The listing builds one solid part. Answer for the finished solid, in the listing's coordinates (mm). A direction names the side the tool comes from. Give positions to 0.01 mm unless a question says otherwise; leave off trailing zeros. Loops run counter-clockwise (first coordinate to the right, second up) from the corner with the lowest first, then second, coordinate; pieces in that order, holes last. Notation, with made-up numbers: (-9.5, -19.5) - (4.5, -19.5) arc R19 cw to (4.5, -4.5) - close; hole circle Ø10 at (29.25, 16). An arc over 180 degrees is marked (long way). Write each question's results on one line, items separated by ' | '.
from build123d import *
from OCP.BRepFilletAPI import BRepFilletAPI_MakeChamfer

# Parameters (mm, degrees)
SKETCH1_W           = 225
SKETCH1_H           = 190
SKETCH1_R           = 2.65
BOSS_EXTRUDE1_DEPTH = 5
BOSS_EXTRUDE2_DEPTH = 5
CHAMFER1_SIZE       = 8.660254038
CHAMFER1_SIZE_2     = 5


with BuildPart() as part:
    # Sketch1 → Boss-Extrude1 (new body)
    with BuildSketch(Plane(origin=(0, 0, 0), x_dir=(1, 0, 0), z_dir=(0, 1, 0))):
        with Locations((112.5, 95)):
            Rectangle(SKETCH1_W, SKETCH1_H)
        with Locations(Location((10, 180, 0), (0, 0, 270))):
            Circle(SKETCH1_R, mode=Mode.SUBTRACT)
        with Locations(Location((40, 180, 0), (0, 0, 270))):
            Circle(SKETCH1_R, mode=Mode.SUBTRACT)
        with Locations(Location((185, 180, 0), (0, 0, 270))):
            Circle(SKETCH1_R, mode=Mode.SUBTRACT)
        with Locations(Location((215, 180, 0), (0, 0, 270))):
            Circle(SKETCH1_R, mode=Mode.SUBTRACT)
        with Locations(Location((215, 10, 0), (0, 0, 90))):
            Circle(SKETCH1_R, mode=Mode.SUBTRACT)
        with Locations(Location((185, 10, 0), (0, 0, 90))):
            Circle(SKETCH1_R, mode=Mode.SUBTRACT)
        with Locations(Location((40, 10, 0), (0, 0, 90))):
            Circle(SKETCH1_R, mode=Mode.SUBTRACT)
        with Locations(Location((10, 10, 0), (0, 0, 90))):
            Circle(SKETCH1_R, mode=Mode.SUBTRACT)
    extrude(amount=BOSS_EXTRUDE1_DEPTH)

    # Sketch2 → Boss-Extrude2 (add)
    with BuildSketch(Plane(origin=(0, 5, 0), x_dir=(1, 0, 0), z_dir=(0, 1, 0))):
        with BuildLine():
            Line((51.576473623, 139.026400418), (167.040167682, 43.276019978))
            ThreePointArc((167.040167682, 43.276019978), (174.080636831, 43.933130432), (173.423526377, 50.973599582))
            Line((173.423526377, 50.973599582), (57.959832318, 146.723980022))
            ThreePointArc((57.959832318, 146.723980022), (50.919363169, 146.066869568), (51.576473623, 139.026400418))
        make_face()
    boss_extrude2 = extrude(amount=BOSS_EXTRUDE2_DEPTH)

    # Mirror1: Boss-Extrude2 across plane
    add(boss_extrude2.mirror(Plane(origin=(0, 0, -95), x_dir=(1, 0, 0), z_dir=(0, 0, -1))))

    # Chamfer1
    chamfer1_edges_1 = [part.edges().sort_by_distance(p)[0] for p in [
        (139.770083841, 5, -65.890235846),
    ]]
    chamfer1_side_1 = [part.faces().sort_by_distance(p)[0] for p in [
        (139.706250254, 5, -65.81326005),
    ]]
    chamfer1_edges_2 = [part.edges().sort_by_distance(p)[0] for p in [
        (174.080636831, 5, -43.933130432),
    ]]
    chamfer1_side_2 = [part.faces().sort_by_distance(p)[0] for p in [
        (174.157612628, 5, -43.869296845),
    ]]
    chamfer1_edges_3 = [part.edges().sort_by_distance(p)[0] for p in [
        (146.878196714, 5, -72.986799791),
    ]]
    chamfer1_side_3 = [part.faces().sort_by_distance(p)[0] for p in [
        (146.942030301, 5, -73.063775587),
    ]]
    chamfer1_edges_4 = [part.edges().sort_by_distance(p)[0] for p in [
        (146.878196714, 5, -117.013200209),
    ]]
    chamfer1_side_4 = [part.faces().sort_by_distance(p)[0] for p in [
        (146.942030301, 5, -116.936224413),
    ]]
    chamfer1_edges_5 = [part.edges().sort_by_distance(p)[0] for p in [
        (174.080636831, 5, -146.066869568),
    ]]
    chamfer1_side_5 = [part.faces().sort_by_distance(p)[0] for p in [
        (174.157612628, 5, -146.130703155),
    ]]
    chamfer1_edges_6 = [part.edges().sort_by_distance(p)[0] for p in [
        (139.770083841, 5, -124.109764154),
    ]]
    chamfer1_side_6 = [part.faces().sort_by_distance(p)[0] for p in [
        (139.706250254, 5, -124.18673995),
    ]]
    chamfer1_edges_7 = [part.edges().sort_by_distance(p)[0] for p in [
        (85.229916159, 5, -124.109764154),
    ]]
    chamfer1_side_7 = [part.faces().sort_by_distance(p)[0] for p in [
        (85.293749746, 5, -124.18673995),
    ]]
    chamfer1_edges_8 = [part.edges().sort_by_distance(p)[0] for p in [
        (85.229916159, 5, -65.890235846),
    ]]
    chamfer1_side_8 = [part.faces().sort_by_distance(p)[0] for p in [
        (85.293749746, 5, -65.81326005),
    ]]
    chamfer1_edges_9 = [part.edges().sort_by_distance(p)[0] for p in [
        (50.919363169, 5, -146.066869568),
    ]]
    chamfer1_side_9 = [part.faces().sort_by_distance(p)[0] for p in [
        (50.842387372, 5, -146.130703155),
    ]]
    chamfer1_edges_10 = [part.edges().sort_by_distance(p)[0] for p in [
        (50.919363169, 5, -43.933130432),
    ]]
    chamfer1_side_10 = [part.faces().sort_by_distance(p)[0] for p in [
        (50.842387372, 5, -43.869296845),
    ]]
    chamfer1_edges_11 = [part.edges().sort_by_distance(p)[0] for p in [
        (78.121803286, 5, -117.013200209),
    ]]
    chamfer1_side_11 = [part.faces().sort_by_distance(p)[0] for p in [
        (78.057969699, 5, -116.936224413),
    ]]
    chamfer1_edges_12 = [part.edges().sort_by_distance(p)[0] for p in [
        (78.121803286, 5, -72.986799791),
    ]]
    chamfer1_side_12 = [part.faces().sort_by_distance(p)[0] for p in [
        (78.057969699, 5, -73.063775587),
    ]]
    chamfer1 = BRepFilletAPI_MakeChamfer(part.part.solid().wrapped)
    for e in chamfer1_edges_1:
        chamfer1.Add(CHAMFER1_SIZE - 0.0001, CHAMFER1_SIZE_2 - 0.0001, e.wrapped, chamfer1_side_1[0].wrapped)
    for e in chamfer1_edges_2:
        chamfer1.Add(CHAMFER1_SIZE - 0.0001, CHAMFER1_SIZE_2 - 0.0001, e.wrapped, chamfer1_side_2[0].wrapped)
    for e in chamfer1_edges_3:
        chamfer1.Add(CHAMFER1_SIZE - 0.0001, CHAMFER1_SIZE_2 - 0.0001, e.wrapped, chamfer1_side_3[0].wrapped)
    for e in chamfer1_edges_4:
        chamfer1.Add(CHAMFER1_SIZE - 0.0001, CHAMFER1_SIZE_2 - 0.0001, e.wrapped, chamfer1_side_4[0].wrapped)
    for e in chamfer1_edges_5:
        chamfer1.Add(CHAMFER1_SIZE - 0.0001, CHAMFER1_SIZE_2 - 0.0001, e.wrapped, chamfer1_side_5[0].wrapped)
    for e in chamfer1_edges_6:
        chamfer1.Add(CHAMFER1_SIZE - 0.0001, CHAMFER1_SIZE_2 - 0.0001, e.wrapped, chamfer1_side_6[0].wrapped)
    for e in chamfer1_edges_7:
        chamfer1.Add(CHAMFER1_SIZE - 0.0001, CHAMFER1_SIZE_2 - 0.0001, e.wrapped, chamfer1_side_7[0].wrapped)
    for e in chamfer1_edges_8:
        chamfer1.Add(CHAMFER1_SIZE - 0.0001, CHAMFER1_SIZE_2 - 0.0001, e.wrapped, chamfer1_side_8[0].wrapped)
    for e in chamfer1_edges_9:
        chamfer1.Add(CHAMFER1_SIZE - 0.0001, CHAMFER1_SIZE_2 - 0.0001, e.wrapped, chamfer1_side_9[0].wrapped)
    for e in chamfer1_edges_10:
        chamfer1.Add(CHAMFER1_SIZE - 0.0001, CHAMFER1_SIZE_2 - 0.0001, e.wrapped, chamfer1_side_10[0].wrapped)
    for e in chamfer1_edges_11:
        chamfer1.Add(CHAMFER1_SIZE - 0.0001, CHAMFER1_SIZE_2 - 0.0001, e.wrapped, chamfer1_side_11[0].wrapped)
    for e in chamfer1_edges_12:
        chamfer1.Add(CHAMFER1_SIZE - 0.0001, CHAMFER1_SIZE_2 - 0.0001, e.wrapped, chamfer1_side_12[0].wrapped)
    add(Compound.cast(chamfer1.Shape()), mode=Mode.REPLACE)  # a hair under: the kernel refuses the full size


solid = part.part
Item 1: A cutting plane is placed at A-A, the plane z = -180. Determine the outline of the cut face in (x, y).
Values found:
outline: (0, 0) - (7.35, 0) - (7.35, 5) - (0, 5) - close; (12.65, 0) - (37.35, 0) - (37.35, 5) - (12.65, 5) - close; (42.65, 0) - (182.35, 0) - (182.35, 5) - (42.65, 5) - close; (187.65, 0) - (212.35, 0) - (212.35, 5) - (187.65, 5) - close; (217.65, 0) - (225, 0) - (225, 5) - (217.65, 5) - close
Item 2: Find the intervals of material crossed by line 1 along X through (y, z) = (2.35, -10); line 2 along Z through (x, y) = (215, 1.15); line 3 along Y through (x, z) = (176, -162), in increasing order. Write a range as [from, to].
Values found:
line 1: x = [0, 7.35], [12.65, 37.35], [42.65, 182.35], [187.65, 212.35], [217.65, 225] | line 2: z = [-190, -182.65], [-177.35, -12.65], [-7.35, 0] | line 3: y = [0, 5]
Item 3: A cutting plane is placed at C-C, the plane y = 8. Determine the outline of the cut face in (x, z).
Values found:
outline: (49.37, -136.36) arc R8.46 ccw to (60.17, -149.39) - (112.5, -106) - (164.83, -149.39) arc R8.46 ccw to (175.63, -136.36) - (125.76, -95) - (175.63, -53.64) arc R8.46 ccw to (164.83, -40.61) - (112.5, -84) - (60.17, -40.61) arc R8.46 ccw to (49.37, -53.64) - (99.24, -95) - close
Item 4: Flat-ended cylindrical pins translate along their axes: P1, Ø5, axis at x = 215, z = -180, coming from the +Y side; P2, Ø7, axis at x = 215, z = -10, coming from the +Y side; P3, Ø6, axis at x = 185, z = -180, coming from the -Y side. Find the tip coordinate at first contact, or state that the pin passes through.
Values found:
P1: passes through | P2: stops at y = 5 | P3: stops at y = 0
Item 5: A cutting plane is placed at B-B, the plane x = 215. Determine the outline of the cut face in (y, z).
Values found:
outline: (0, -190) - (5, -190) - (5, -182.65) - (0, -182.65) - close; (0, -177.35) - (5, -177.35) - (5, -12.65) - (0, -12.65) - close; (0, -7.35) - (5, -7.35) - (5, 0) - (0, 0) - close
Item 6: For faces 5 (the face through (88.337, 7.535, -127.08)), 6 (the face through (111, 5, -75)), 7 (the face through (40.796, 2.465, -177.472)), determine the directions among +Z, -Z, +X, -X, +Y, -Y from which every point of the face is accessible in a straight line to the end or side of a thin tool.
Values found:
face 5: -Z, +Y | face 6: +Y | face 7: +Y, -Y
Item 7: For a pull along X with two mould halves and no side action, classify faces 1 (the face through (225, 2, -94)), 2 (the face through (182.37, 2.46, -9.66)), 3 (the face through (112, 10, -95)), 4 (the face through (49.95, 9.2, -42.94)) as released by +X, released by -X, zero draft, split by the parting line, or undercut.
Values found:
face 1: released by +X | face 2: undercut | face 3: zero draft | face 4: undercut
